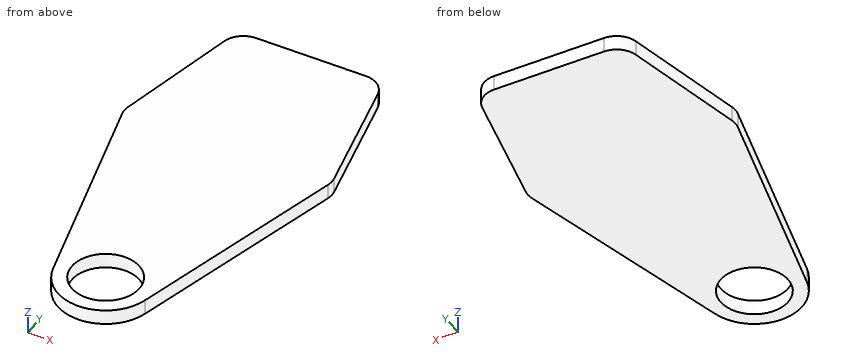
from build123d import *

# Parameters (mm, degrees)
SKETCH1_R           = 15.24
BOSS_EXTRUDE1_DEPTH = 6.731
FILLET1_R           = 10.16
FILLET2_R           = 10.16


with BuildPart() as part:
    # Sketch1 → Boss-Extrude1 (new body)
    with BuildSketch(Plane.XY):
        with BuildLine():
            Line((-33.2359, 164.676666667), (33.2359, 164.676666667))
            Line((33.2359, 164.676666667), (47.4853, 98.171))
            Line((47.4853, 98.171), (20.912246435, -5.367126704))
            ThreePointArc((20.912246435, -5.367126704), (0, -21.59), (-20.912246435, -5.367126704))
            Line((-20.912246435, -5.367126704), (-47.4853, 98.171))
            Line((-47.4853, 98.171), (-33.2359, 164.676666667))
        make_face()
        Circle(SKETCH1_R, mode=Mode.SUBTRACT)
    extrude(amount=BOSS_EXTRUDE1_DEPTH)

    # Fillet1
    fillet1_edges = [part.edges().sort_by_distance(p)[0] for p in [
        (-47.4853, 98.171, 3.3655),
        (47.4853, 98.171, 3.3655),
    ]]
    fillet(fillet1_edges, radius=FILLET1_R)

    # Fillet2
    fillet2_edges = [part.edges().sort_by_distance(p)[0] for p in [
        (-33.2359, 164.676666667, 3.3655),
        (33.2359, 164.676666667, 3.3655),
    ]]
    fillet(fillet2_edges, radius=FILLET2_R)


solid = part.part
Geometry check sheet. Reference: the model listing, model coordinates, mm. Round coordinates to 2 decimals unless told otherwise and drop trailing zeros. Write each loop counter-clockwise with the first axis right and the second up, starting at its lowest first coordinate (ties: lowest second). Pieces come first, ordered by that corner, then holes.
Item 1: Section check A-A (x = 0). Record the boundary of the cut face in (y, z).
Determined:
outline: (-21.59, 0) - (-15.24, 0) - (-15.24, 6.73) - (-21.59, 6.73) - close; (15.24, 0) - (164.68, 0) - (164.68, 6.73) - (15.24, 6.73) - close
Item 2: Section check B-B (z = 2.75). Record the boundary of the cut face in (x, y).
Determined:
outline: (-46.98, 100.51) arc R10.16 ccw to (-46.89, 95.85) - (-20.91, -5.37) arc R21.59 ccw to (20.91, -5.37) - (46.89, 95.85) arc R10.16 ccw to (46.98, 100.51) - (34.96, 156.65) arc R10.16 ccw to (25.02, 164.68) - (-25.02, 164.68) arc R10.16 ccw to (-34.96, 156.65) - close; hole circle Ø30.48 at (0, 0)
Item 3: Material ranges on line 1 along Y through (x, z) = (0, 3.75); line 2 along Y through (x, z) = (6, 1); line 3 along X through (y, z) = (1.5, 3.5), recorded low to high.
Determined:
line 1: y = -21.59 to -15.24, 15.24 to 164.68
line 2: y = -20.74 to -14.01, 14.01 to 164.68
line 3: x = -22.67 to -15.17, 15.17 to 22.67
Item 4: Go/stop test with flat-tipped pins: pin 1 Ø18.5 at (x, y) = (0, 0) entering from +Z; pin 2 Ø12 at (x, y) = (7, 123) entering from -Z; pin 3 Ø2 at (y, z) = (62, 3) entering from -X. Record where each tip stops, or that it passes through.
Determined:
pin 1: passes through
pin 2: stops at z = 0
pin 3: stops at x = -38.46
Item 5: Section check D-D (y = 53.5). Record the boundary of the cut face in (x, z).
Determined:
outline: (-36.02, 0) - (36.02, 0) - (36.02, 6.73) - (-36.02, 6.73) - close
Item 6: Section check C-C (y = 7). Record the boundary of the cut face in (x, z), plus the area to 3 significant figures.
Determined:
outline: (-24.09, 0) - (-13.54, 0) - (-13.54, 6.73) - (-24.09, 6.73) - close; (13.54, 0) - (24.09, 0) - (24.09, 6.73) - (13.54, 6.73) - close
area: 142 mm2
